The model under review builds one solid part; all positions refer to its coordinate system, in mm. Face numbers are marked on the shaded views. A direction names the side the tool comes from. Coordinates: 2 decimals unless noted, no trailing zeros. Order: outer loops, then holes, each group sorted by start corner. A loop starts at its lowest first (then second) coordinate and runs counter-clockwise, first axis right, second up. Notation, with made-up numbers: (4.5, 47.5) - (62.5, 47.5) arc R18 ccw to (62.5, 63.5) - close; hole circle Ø2 at (20.25, 58). An arc over 180 degrees is marked (long way). Answer in a Markdown table with one row per item.
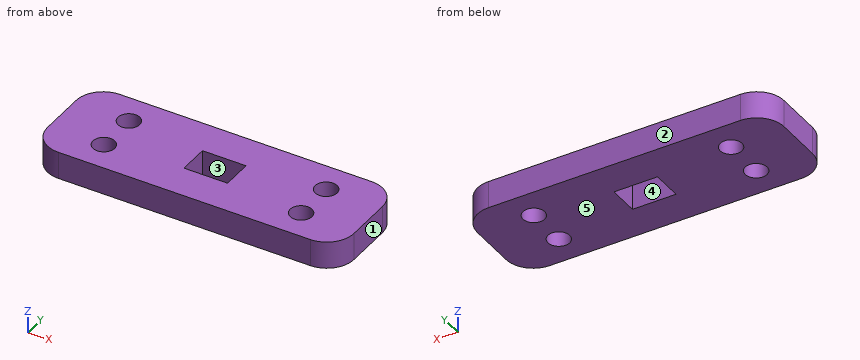
Autodesk Inventor part; units mm, degrees
ref_plane "Work Plane1" through (35.7251, -23.622, 0) normal (1, 0, 0) x (0, 0, -1)
ref_plane "YZ Plane" through (0, 0, 0) normal (1, 0, 0) x (0, 1, 0)
ref_plane "XZ Plane" through (0, 0, 0) normal (0, 1, 0) x (-1, 0, 0)
sketch "Sketch1" plane through (0, 0, 0) normal (0, 0, 1) x (1, 0, 0)
  line L0 (0, 0) -> (71.4502, 0)
  line L1 (71.4502, 0) -> (71.4502, -23.622)
  line L2 (71.4502, -23.622) -> (0, -23.622)
  line L3 (0, -23.622) -> (0, 0)
  dimension "d0" = 71.4502
  dimension "d1" = 23.622
extrude "Extrusion1" add sketch "Sketch1" along normal blind 6.35
sketch "Sketch3" plane through (0, 0, 6.35) normal (0, 0, 1) x (1, 0, 0)
  line L0 (0, -23.622) -> (71.4502, -23.622)
  line L1 (71.4502, 0) -> (0, 0)
  line L2 (71.4502, -23.622) -> (71.4502, 0)
  point P0 (58.7248, -6.985)
  point P1 (58.7248, -16.637)
  dimension "d15" = 6.985
  dimension "d16" = 6.985
  dimension "d17" = 12.7254
  dimension "d18" = 12.7254
hole "Hole2" at (58.7248, -6.985, 6.35) at (58.7248, -16.637, 6.35) direction (0, 0, -1) diameter 5.08 depth 25.4 tip angle 118
ref_plane "Work Plane1" through (35.7251, -23.622, 0) normal (1, 0, 0) x (0, 0, -1)
mirror "Mirror1" about plane through (35.7251, -23.622, 0) normal (1, 0, 0) of "Hole2"
sketch "Sketch4" plane through (0, 0, 6.35) normal (0, 0, 1) x (1, 0, 0)
  line L0 (30.6451, -8.255) -> (40.8051, -8.255)
  line L1 (40.8051, -8.255) -> (40.8051, -15.367)
  line L2 (40.8051, -15.367) -> (30.6451, -15.367)
  line L3 (30.6451, -15.367) -> (30.6451, -8.255)
  line L4 (71.4502, -23.622) -> (71.4502, 0)
  line L5 (0, 0) -> (0, -23.622)
  line L6 (71.4502, 0) -> (0, 0)
  line L7 (0, -23.622) -> (71.4502, -23.622)
  dimension "d26" = 10.16
  dimension "d27" = 7.112
  dimension "d28" = 71.4502
  dimension "d29" = 30.6451
  dimension "d30" = 8.255
  dimension "d31" = 23.622
extrude "Extrusion2" cut sketch "Sketch4" against normal blind 6.35 contours L0 L1 L2 L3
fillet "Fillet1" radius 6.35 4 edges at (71.4502, 0, 3.175) (71.4502, -23.622, 3.175) (0, 0, 3.175) (0, -23.622, 3.175)
properties part number "phone cord holder"
Item 1: To check wall thickness, follow line 1 (Y direction, x = 12.5, z = 6); line 2 (X direction, y = -16.75, z = 3.5); line 3 (Y direction, x = 14.5, z = 3.5). State the ranges of each line that lie inside material, in increasing order. Write a range as from..to.
Check values:
| item | result |
|---|---|
| line 1 | -23.62..-19.17, -14.11..-9.51, -4.46..0 |
| line 2 | 0..10.19, 15.26..56.19, 61.26..71.45 |
| line 3 | -23.62..-18.45, -14.82..-8.8, -5.17..0 |
Item 2: We need section B-B, the plane y = -11. Write out the cut boundary in (x, z), then the cut area to 3 significant figures.
Check values:
| item | result |
|---|---|
| outline | (0, 0) - (30.65, 0) - (30.65, 6.35) - (0, 6.35) - close; (40.81, 0) - (71.45, 0) - (71.45, 6.35) - (40.81, 6.35) - close |
| area | 389 mm^2 |
Item 3: Mouldability with a two-part tool opening along Y and no side actions: class the marked faces 1, 2 and 3 as +Y half, -Y half, draft (parallel to the pull), parting line (faces both ways), or undercut.
Check values:
| item | result |
|---|---|
| face 1 | draft |
| face 2 | +Y half |
| face 3 | undercut |
Item 4: Tool access review of the marked faces 4 and 5: name each direction out of +Z, -Z, +X, -X, +Y, -Y from which nothing blocks a thin tool from reaching the whole face with its end or side.
Check values:
| item | result |
|---|---|
| face 4 | +Z, -Z |
| face 5 | -Z, +X, -X, +Y, -Y |
Item 5: We need section D-D, the plane x = 14. Write out the cut boundary in (y, z).
Check values:
| item | result |
|---|---|
| outline | (-23.62, 0) - (-18.83, 0) - (-18.83, 6.35) - (-23.62, 6.35) - close; (-14.44, 0) - (-9.18, 0) - (-9.18, 6.35) - (-14.44, 6.35) - close; (-4.79, 0) - (0, 0) - (0, 6.35) - (-4.79, 6.35) - close |
Item 6: Clearance check with a flat-ended pin moving along its axis: pin 1 Ø1.5 at (y, z) = (-20, 4) entering from +X. State where the tip first meets the part, or that it passes through.
Check values:
| item | result |
|---|---|
| pin 1 | x = 71.13 |
Item 7: We need section A-A, the plane x = 32. Write out the cut boundary in (y, z) (3 decimals).
Check values:
| item | result |
|---|---|
| outline | (-23.622, 0) - (-15.367, 0) - (-15.367, 6.35) - (-23.622, 6.35) - close; (-8.255, 0) - (0, 0) - (0, 6.35) - (-8.255, 6.35) - close |
Item 8: We need section C-C, the plane z = 4. Write out the cut boundary in (x, y) (3 decimals), then the cut area to 3 significant figures.
Check values:
| item | result |
|---|---|
| outline | (0, -17.272) arc R6.35 ccw to (6.35, -23.622) - (65.1, -23.622) arc R6.35 ccw to (71.45, -17.272) - (71.45, -6.35) arc R6.35 ccw to (65.1, 0) - (6.35, 0) arc R6.35 ccw to (0, -6.35) - close; hole circle Ø5.08 at (12.725, -16.637); hole circle Ø5.08 at (12.725, -6.985); hole (30.645, -15.367) - (40.805, -15.367) - (40.805, -8.255) - (30.645, -8.255) - close; hole circle Ø5.08 at (58.725, -16.637); hole circle Ø5.08 at (58.725, -6.985) |
| area | 1,500 mm^2 |
